Model file for the job. Use its own axes, mm. A direction names the side the tool comes from. Give positions to 0.01 mm unless a question says otherwise; leave off trailing zeros. Loops run counter-clockwise (first coordinate to the right, second up) from the corner with the lowest first, then second, coordinate; pieces in that order, holes last. Notation, with made-up numbers: M 62,62.25 L 80,62.25 A26 cw 80,95.25 Z; hole C 21,-12 d11. An arc over 180 degrees is marked long. Answer in a Markdown table with one row per item.
Autodesk Inventor part; units mm, degrees
ref_plane "Work Plane1" through (0, 12.4, 0) normal (0, 1, 0) x (1, 0, 0)
ref_plane "YZ Plane" through (0, 0, 0) normal (1, 0, 0) x (0, 1, 0)
ref_plane "XZ Plane" through (0, 0, 0) normal (0, 1, 0) x (-1, 0, 0)
sketch "Sketch1" plane through (0, 0, 0) normal (0, 1, 0) x (-1, 0, 0)
  circle A0 centre (0, 0) radius 20.5
  dimension "d0" = 41
extrude "Extrusion1" add sketch "Sketch1" along normal blind 20.4
sketch "Sketch2" plane through (0, 20.4, 0) normal (0, 1, 0) x (1, 0, 0)
  line L0 (-25.2236, 0) -> (25.6343, 0)
  circle A0 centre (0, 0) radius 17.2 construction
  point P0 (-17.2, 0)
  point P1 (8.6, -14.8956)
  point P2 (8.6, 14.8956)
  dimension "d3" = 34.4
  dimension "d6" = 360
hole "Hole1" at (-17.2, 20.4, 0) at (8.6, 20.4, 14.8956) at (8.6, 20.4, -14.8956) direction (0, -1, 0) diameter 3 end through all counterbore diameter 4.4 counterbore depth 2
sketch "Sketch3" plane through (0, 20.4, 0) normal (0, 1, 0) x (1, 0, 0)
  circle A0 centre (8.6, -14.8956) radius 2.2
  circle A1 centre (-17.2, 0) radius 2.2
  circle A2 centre (8.6, 14.8956) radius 2.2
  circle A3 centre (0, 0) radius 20.5
  line L0 (6.5697, -15.7429) -> (7.895, -18.9187)
  circle A4 centre (0, 0) radius 20.5
  line L1 (10.3489, -13.561) -> (12.4366, -16.2966)
  line L2 (10.3489, 13.561) -> (12.4366, 16.2966)
  line L3 (6.5697, 15.7429) -> (7.895, 18.9187)
  line L4 (-16.9186, 2.1819) -> (-20.3316, 2.6221)
  line L5 (-16.9186, -2.1819) -> (-20.3316, -2.6221)
  circle A5 centre (-17.2, 0) radius 2.2
  circle A6 centre (8.6, 14.8956) radius 2.2
  circle A7 centre (8.6, -14.8956) radius 2.2
extrude "Extrusion2" cut sketch "Sketch3" against normal blind 2 contours A0 L1 A3 L0 | A3 L4 A1 L5 | L2 A2 L3 A3
ref_plane "Work Plane1" through (0, 12.4, 0) normal (0, 1, 0) x (1, 0, 0)
sketch "Sketch4" plane through (0, 12.4, 0) normal (0, 1, 0) x (1, 0, 0)
  circle A0 centre (8.6, -14.8956) radius 1.5
  circle A1 centre (-17.2, 0) radius 1.5
  circle A2 centre (8.6, 14.8956) radius 1.5
  circle A3 centre (0, 0) radius 20.5
  line L0 (0, 0) -> (-21.2105, -12.2459) construction
  line L1 (0, 0) -> (-21.8671, 12.625) construction
  line L2 (-23.6336, 0) -> (24.9961, 0) construction
  line L3 (0, 0) -> (0, -27.2781) construction
  line L4 (-12.9995, 7.5053) -> (-21.8671, 12.625) construction
  line L5 (-12.3745, 8.5878) -> (-21.2421, 13.7075)
  line L6 (-22.4921, 11.5425) -> (-13.6245, 6.4228)
  arc A4 (-13.6245, 6.4228) -> (-12.3745, 8.5878) centre (-12.9995, 7.5053) ccw
  arc A5 (-21.2421, 13.7075) -> (-22.4921, 11.5425) centre (-21.8671, 12.625) ccw
  line L7 (-21.8671, -12.625) -> (-13.5975, -7.8505) construction
  line L8 (-21.2421, -13.7075) -> (-12.9725, -8.9331)
  line L9 (-14.2225, -6.768) -> (-22.4921, -11.5425)
  arc A6 (-22.4921, -11.5425) -> (-21.2421, -13.7075) centre (-21.8671, -12.625) ccw
  arc A7 (-12.9725, -8.9331) -> (-14.2225, -6.768) centre (-13.5975, -7.8505) ccw
  line L10 (0, -25.25) -> (0, -15.6538) construction
  line L11 (1.25, -25.25) -> (1.25, -15.6538)
  line L12 (-1.25, -15.6538) -> (-1.25, -25.25)
  arc A8 (-1.25, -25.25) -> (1.25, -25.25) centre (0, -25.25) ccw
  arc A9 (1.25, -15.6538) -> (-1.25, -15.6538) centre (0, -15.6538) ccw
  point P0 (-17.4333, 10.0651)
  point P1 (-17.7323, -10.2378)
  point P2 (0, -20.4519)
  point P3 (-18.3455, 9.1484)
  point P4 (-17.0955, 11.3135)
  dimension "d18" = 30
  dimension "d19" = 30
  dimension "d20" = 60
  dimension "d21" = 2.5
  dimension "d22" = 6
  dimension "d23" = 2.5
  dimension "d24" = 2.5
  dimension "d25" = 6
  dimension "d26" = 6
extrude "Extrusion3" add sketch "Sketch4" against normal blind 0.5 contours A3 L6 A5 L5 | L11 A8 L12 A3 | A3 L12 A9 L11 | L9 A7 L8 A3 | A3 L8 A6 L9
sketch "Sketch5" plane through (0, 0, 0) normal (0, -1, 0) x (1, 0, 0)
  arc A0 (-17.0955, 11.3135) -> (-18.3455, 9.1484) centre (0, 0) ccw
  line L0 (-17.0955, 11.3135) -> (-21.2421, 13.7075)
  arc A1 (-21.2421, 13.7075) -> (-22.4921, 11.5425) centre (-21.8671, 12.625) ccw
  line L1 (-22.4921, 11.5425) -> (-18.3455, 9.1484)
  line L2 (-18.3455, -9.1484) -> (-22.4921, -11.5425)
  arc A2 (-22.4921, -11.5425) -> (-21.2421, -13.7075) centre (-21.8671, -12.625) ccw
  line L3 (-21.2421, -13.7075) -> (-17.0955, -11.3135)
  arc A3 (-18.3455, -9.1484) -> (-17.0955, -11.3135) centre (0, 0) ccw
  arc A4 (1.25, 20.4619) -> (-1.25, 20.4619) centre (0, 0) ccw
  line L4 (1.25, 20.4619) -> (1.25, 25.25)
  arc A5 (1.25, 25.25) -> (-1.25, 25.25) centre (0, 25.25) ccw
  line L5 (-1.25, 25.25) -> (-1.25, 20.4619)
  circle A6 centre (8.6, 14.8956) radius 1.5
  circle A7 centre (-17.2, 0) radius 1.5
  circle A8 centre (8.6, -14.8956) radius 1.5
  circle A9 centre (0, 0) radius 20.5
  line L6 (0, 34.5014) -> (0, -27.9837) construction
  line L7 (0, 0) -> (-32.677, 18.8661) construction
  line L8 (0, 0) -> (-32.677, -18.8661) construction
  circle A10 centre (0, 0) radius 17.2 construction
  circle A11 centre (0, 17.2) radius 1.5
  circle A12 centre (-14.8956, 8.6) radius 1.5
  circle A13 centre (-14.8956, -8.6) radius 1.5
  dimension "d29" = 34.4
  dimension "d30" = 3
  dimension "d31" = 3
  dimension "d32" = 3
extrude "Extrusion4" cut sketch "Sketch5" against normal blind 0.2 contours A11 | A12 | A13
sketch "Sketch7" plane through (-14.8956, 0.2, 8.6) normal (0, -1, 0) x (1, 0, 0)
  circle A0 centre (14.8956, 8.6) radius 1.5
  circle A1 centre (0, 0) radius 1.5
  circle A2 centre (0, -17.2) radius 1.5
  circle A3 centre (23.4956, 6.2956) radius 1.5
  circle A4 centre (-2.3044, -8.6) radius 1.5
  circle A5 centre (23.4956, -23.4956) radius 1.5
  circle A6 centre (14.8956, -8.6) radius 20.5
  circle A7 centre (0, 0) radius 0.5
  circle A8 centre (14.8956, 8.6) radius 0.5
  circle A9 centre (0, -17.2) radius 0.5
  dimension "d36" = 1
  dimension "d37" = 1
  dimension "d38" = 1
extrude "Extrusion5" add sketch "Sketch7" along normal blind 4.5 contours A7 | A8 | A9
fillet "Fillet1" radius 0.5 3 edges at (-15.3956, -4.3, -8.6) (-15.3956, -4.3, 8.6) (-0.5, -4.3, 17.2)
fillet "Fillet2" radius 1 4 edges at (-10.25, 20.4, 17.7535) (-10.25, 20.4, -17.7535) (20.5, 20.4, 0) (20.5, 0, 0)
properties part number "S200 EChem Sensor"
Q1. Drop flat-ended pins along their axis: pin 1 (0.8 mm diameter, centred on x = 0.5, z = 24.5, fed in from +Y); pin 2 (4 mm diameter, centred on x = 12.5, z = 16.5, fed in from -Y); pin 3 (0.9 mm diameter, centred on x = -15.5, z = 9, fed in from -Y). Give the stop position or say it passes through.
Reported:
| item | result |
|---|---|
| pin 1 | y = 12.4 |
| pin 2 | y = 0 |
| pin 3 | y = -4.22 |
Q2. Probe probe 1 along Z at (x, y) = (8.6, 9); probe 2 along Y at (x, z) = (6.5, -11); probe 3 along X at (y, z) = (0.5, 14.5). List the from-to ranges inside material, lowest first.
Reported:
| item | result |
|---|---|
| probe 1 | -18.61 to -16.4, -13.4 to 13.4, 16.4 to 18.61 |
| probe 2 | 0 to 20.4 |
| probe 3 | -14.3 to 7.15, 10.05 to 14.3 |
Q3. Saw through at D-D (x = 8.6). Give the number of separate pieces and of enclosed holes in the cut face, and give its area (3 significant figures).
Reported:
| item | result |
|---|---|
| separate pieces | 3 |
| enclosed holes | 0 |
| area | 625 mm² |
Q4. Mould opens along X. For faces 1 (the face through (-20.39, 12.15, 10.33)), 2 (the face through (-20, 12.4, 11)), 3 (the face through (7.223, 19.414, -17.309)) say: released by +X, released by -X, zero draft, split by the parting line, or undercut.
Reported:
| item | result |
|---|---|
| face 1 | released by -X |
| face 2 | zero draft |
| face 3 | undercut |
Q5. Saw through at B-B (y = 10.25). Give the cut face in (x, z), and give its area (3 significant figures).
Reported:
| item | result |
|---|---|
| outline | C 0,0 d41; hole C -17.2,0 d3; hole C 8.6,-14.9 d3; hole C 8.6,14.9 d3 |
| area | 1,300 mm² |
Q6. Saw through at C-C (y = -2.5). Give the cut face in (x, z), and give its area (3 significant figures).
Reported:
| item | result |
|---|---|
| outline | C -14.9,-8.6 d1; C -14.9,8.6 d1; C 0,17.2 d1 |
| area | 2.36 mm² |
Q7. 3-axis set-ups, long thin cutter, end or side, ignore diameter. For faces 4 (the face through (0, 0.2, 18)), 5 (the face through (-19.14, 12.154, -12.494)), 6 (the face through (-20, 11.9, 11)), 7 (the face through (11.38, 19.41, -14.91)), 8 (the face through (9.4, 18.4, 16.5)): which of +Z, -Z, +X, -X, +Y, -Y reach the whole face in a straight line?
Reported:
| item | result |
|---|---|
| face 4 | -Y |
| face 5 | -Z, +Y, -Y |
| face 6 | +Z, -X, -Y |
| face 7 | -Z, +Y |
| face 8 | +Y |
Q8. Saw through at A-A (z = 0). Give the cut face in (x, y).
Reported:
| item | result |
|---|---|
| outline | M -20.5,1 A1 ccw -19.5,0 L -18.7,0 L -18.7,18.4 L -20.5,18.4 Z; M -15.7,0 L 19.5,0 A1 ccw 20.5,1 L 20.5,19.4 A1 ccw 19.5,20.4 L -15,20.4 L -15,18.4 L -15.7,18.4 Z |
